Print and shaded views of the part. All mm, measured from the part's lowest x, y and z. Round coordinates to 2 decimals unless told otherwise and drop trailing zeros. Loops run counter-clockwise (first coordinate to the right, second up) from the corner with the lowest first, then second, coordinate; pieces in that order, holes last. Notation, with made-up numbers: (35.5, 87) -> (90.5, 87) arc R18 ccw to (90.5, 111) -> close; hole circle Ø11 at (20, 8.25). An arc over 180 degrees is marked (long way). Answer as CSV lines item,"result".
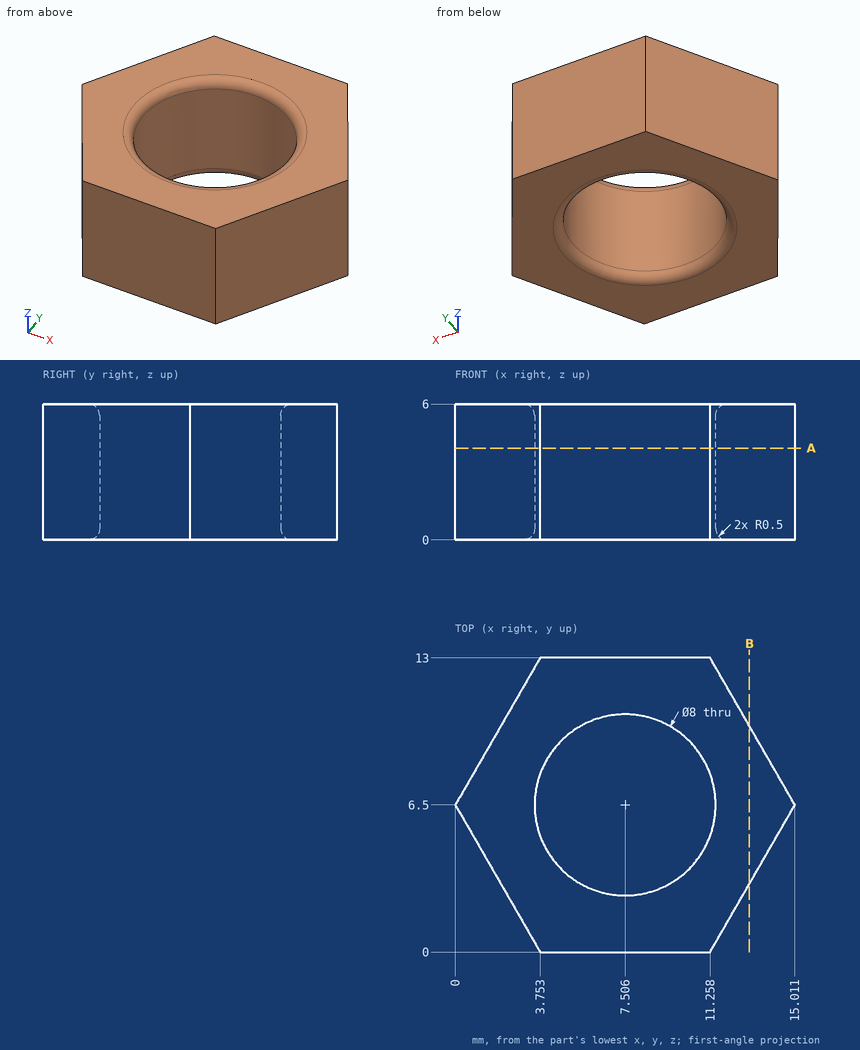
Q1. Saw through at B-B, the plane x = 13. Write the cut outline in (y, z).
Geometry results:
outline,"(3.02, 0) -> (9.98, 0) -> (9.98, 6) -> (3.02, 6) -> close"
Q2. Saw through at A-A, the plane z = 4.05. Write the cut outline in (x, y) (1 decimal).
Geometry results:
outline,"(0, 6.5) -> (3.8, 0) -> (11.3, 0) -> (15, 6.5) -> (11.3, 13) -> (3.8, 13) -> close; hole circle Ø8 at (7.5, 6.5)"
Q3. Drill centre lines: line 1 along Y through (x, z) = (7, 4.2); line 2 along X through (y, z) = (5, 0.7) (1 decimal); line 3 along X through (y, z) = (3.75, 3.55) (1 decimal). Where is each one in solid material? Low to high.
Geometry results:
line 1,"0 to 2.53, 10.47 to 13"
line 2,"0.9 to 3.8, 11.2 to 14.1"
line 3,"1.6 to 4.6, 10.4 to 13.4"
Q4. Drop a flat-ended pin along its axis: P1, Ø1, axis at y = 8, z = 4.5, coming from the +X side (1 decimal). Give the stop position or say it passes through.
Geometry results:
P1,"x = 14.4"
